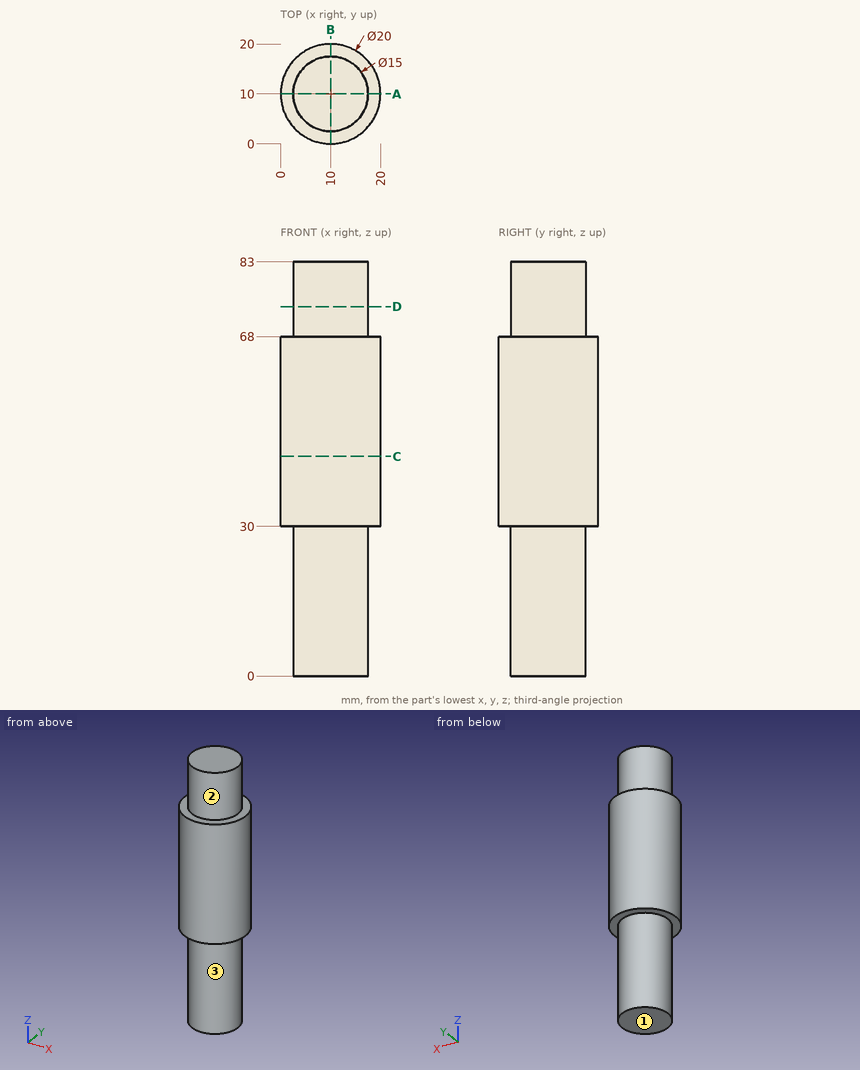
Design review of the part shown in the three views and the two pictorial views. Dimensions are in mm from the part's minimum x, y and z. A direction names the side the tool comes from. Coordinates: 2 decimals unless noted, no trailing zeros. Write each loop counter-clockwise with the first axis right and the second up, starting at its lowest first coordinate (ties: lowest second). Pieces come first, ordered by that corner, then holes. Notation, with made-up numbers: (-25, 33) -> (26, 33) arc R20 cw to (26, 53) -> close; hole circle Ø6 at (16, 60). An arc over 180 degrees is marked (long way). Answer in a Markdown table with one row per item.
1. We need section A-A, the plane y = 10. State the section outline as (x, z) points, and give its area (4 significant figures).
Answers below:
| item | result |
|---|---|
| outline | (0, 30) -> (2.5, 30) -> (2.5, 0) -> (17.5, 0) -> (17.5, 30) -> (20, 30) -> (20, 68) -> (17.5, 68) -> (17.5, 83) -> (2.5, 83) -> (2.5, 68) -> (0, 68) -> close |
| area | 1,435 mm^2 |
2. We need section C-C, the plane z = 44. State the section outline as (x, y) points, and give its area (3 significant figures).
Answers below:
| item | result |
|---|---|
| outline | circle Ø20 at (10, 10) |
| area | 314 mm^2 |
3. We need section D-D, the plane z = 74. State the section outline as (x, y) points.
Answers below:
| item | result |
|---|---|
| outline | circle Ø15 at (10, 10) |
4. Wall thickness on probe 1 along Y at (x, z) = (10.25, 75.5); probe 2 along Z at (x, y) = (3.25, 4): over which ranges is each line inside the solid? List them lowest first. Write a range as [from, to].
Answers below:
| item | result |
|---|---|
| probe 1 | y = [2.5, 17.5] |
| probe 2 | z = [30, 68] |
5. For the marked faces 1, 2 and 3, list the 3-axis set-ups (+Z, -Z, +X, -X, +Y, -Y) from which the entire face can be reached by the end or side of a thin tool; tool diameter is ignored.
Answers below:
| item | result |
|---|---|
| face 1 | -Z, +X, -X, +Y, -Y |
| face 2 | +Z |
| face 3 | -Z |
6. Clearance check with flat-ended pins moving along their axes: pin 1 Ø6 at (y, z) = (15, 73.5) entering from +X; pin 2 Ø8 at (x, z) = (3.5, 44) entering from -Y; pin 3 Ø1.5 at (y, z) = (16.5, 47.5) entering from -X. State where each tip first meets the part, or that it passes through.
Answers below:
| item | result |
|---|---|
| pin 1 | stops at x = 17.23 |
| pin 2 | stops at y = 0.32 |
| pin 3 | stops at x = 1.82 |
